For this review, take the finished solid that the model builds, in its own axes (mm). Coordinates: 2 decimals unless noted, no trailing zeros. Loops run counter-clockwise (first coordinate to the right, second up) from the corner with the lowest first, then second, coordinate; pieces in that order, holes last. Notation, with made-up numbers: (27.25, 35) - (50.25, 35) arc R3 ccw to (50.25, 39) - close; hole circle Ø1 at (11.25, -22). An arc over 180 degrees is marked (long way). Answer as a JSON object with one key per item and string values. Group by question number.
Item 1: To check wall thickness, follow line 1 (X direction, y = -70.5, z = 58); line 2 (Y direction, x = 49.5, z = 7); line 3 (X direction, y = -74, z = 63). State the ranges of each line that lie inside material, in increasing order.
Item 2: Mouldability with a two-part tool opening along Y and no side actions: class faces 1 (the cylindrical face through (74.08, -51.34, 35.16)), 2 (the flat face through (53, 0, 34)), 3 (the flat face through (53, -44, 69.342)), 4 (the cylindrical face through (94.51, -102.63, 35.16)) as released by +Y, released by -Y, zero draft, split by the parting line, or undercut.
Item 3: We need section D-D (y = -99). Give the boundary of the cut face in (x, z).
Item 4: We need section B-B (x = 51). Give the boundary of the cut face in (y, z).
Item 5: We need section A-A (y = -86). Give the boundary of the cut face in (x, z).
Item 6: We need section C-C (z = 45). Give the boundary of the cut face in (x, y), then the cut area to 3 significant figures.
from build123d import *

# Parameters (mm, degrees)
F0_W     = 108.33516
F0_H     = 115.749128
F1_DEPTH = 69.342
F2_R     = 45.990768
F3_R     = 21.838167
F4_DEPTH = 89.916


with BuildPart() as f1:
    # F0 (on Top) → F1 (new body)
    with BuildSketch(Plane.XY):
        with Locations((54.16758, -57.874564)):
            Rectangle(F0_W, F0_H)
    extrude(amount=F1_DEPTH)

    # F2
    f2_edges = [f1.edges().sort_by_distance(p)[0] for p in [
        (108.33516, -115.749128, 34.671),
    ]]
    fillet(f2_edges, radius=F2_R)

    # F3 (on face) → F4 (cut)
    with BuildSketch(Plane.XY.offset(69.342)):
        with Locations((62.344391, -69.75836)):
            Circle(F3_R)
    extrude(amount=-F4_DEPTH, mode=Mode.SUBTRACT)


solid = f1.part
Check sheet entries:
{
 "1": {"line 1": "x = 0 to 40.52, 84.17 to 108.33", "line 2": "y = -115.75 to -87.42, -52.1 to 0", "line 3": "x = 0 to 40.92, 83.77 to 108.14"},
 "2": {"face 1": "undercut", "face 2": "released by +Y", "face 3": "zero draft", "face 4": "released by -Y"},
 "3": {"outline": "(0, 0) - (97.84, 0) - (97.84, 69.34) - (0, 69.34) - close"},
 "4": {"outline": "(-115.75, 0) - (-88.42, 0) - (-88.42, 69.34) - (-115.75, 69.34) - close; (-51.1, 0) - (0, 0) - (0, 69.34) - (-51.1, 69.34) - close"},
 "5": {"outline": "(0, 0) - (47.75, 0) - (47.75, 69.34) - (0, 69.34) - close; (76.94, 0) - (105.37, 0) - (105.37, 69.34) - (76.94, 69.34) - close"},
 "6": {"outline": "(0, -115.75) - (62.34, -115.75) arc R45.99 ccw to (108.34, -69.76) - (108.34, 0) - (0, 0) - close; hole circle Ø43.68 at (62.34, -69.76)", "area": "10,600 mm2"}
}
